Model file for the job. Use its own axes, mm. Face numbers are marked on the shaded views. Coordinates: 2 decimals unless noted, no trailing zeros. Order: outer loops, then holes, each group sorted by start corner. A loop starts at its lowest first (then second) coordinate and runs counter-clockwise, first axis right, second up.
from build123d import *

# Parameters (mm, degrees)
F0_R     = 27
F0_R_2   = 24.925
F1_DEPTH = 13
F0_R_3   = 22.25
F2_DEPTH = 3.5
F3_START = 2.3
F0_R_4   = 27.825
F3_DEPTH = 8.7
F4_SIZE  = 0.3
F5_SIZE  = 0.75


with BuildPart() as f1:
    # F0 (on Top) → F1 (new body)
    with BuildSketch(Plane.XY):
        Circle(F0_R)
        Circle(F0_R_2, mode=Mode.SUBTRACT)
    extrude(amount=F1_DEPTH)

    # F0 (on Top) → F2 (join)
    with BuildSketch(Plane.XY):
        Circle(F0_R_2)
        Circle(F0_R_3, mode=Mode.SUBTRACT)
    extrude(amount=F2_DEPTH)

    # F0 (on Top) → F3 (join)
    with BuildSketch(Plane.XY.offset(F3_START)):
        Circle(F0_R_4)
        Circle(F0_R, mode=Mode.SUBTRACT)
    extrude(amount=F3_DEPTH)

    # F4
    f4_edges = [f1.edges().sort_by_distance(p)[0] for p in [
        (-27, 0, 13),
        (-27, 0, 0),
    ]]
    chamfer(f4_edges, length=F4_SIZE)

    # F5
    f5_edges = [f1.edges().sort_by_distance(p)[0] for p in [
        (27.825, 0, 6.65),
        (-27.825, 0, 2.3),
        (-27.825, 0, 11),
    ]]
    chamfer(f5_edges, length=F5_SIZE)


solid = f1.part
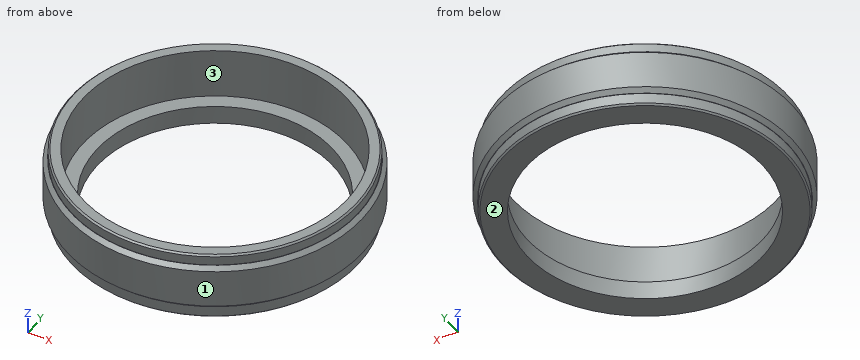
Q1. Mould opens along Y. For the marked faces 1, 2 and 3 say: pulls with the +Y half, pulls with the -Y half, needs draft (parallel to the pull), parting line crosses it, or undercut.
Established:
face 1: parting line crosses it
face 2: needs draft
face 3: undercut
Q2. Probe line 1 (Y direction, x = 0, z = 1.35); line 2 (Y direction, x = 0, z = 8.75) (3 decimals); line 3 (X direction, y = 0.5, z = 9). List the from-to ranges inside material, lowest first.
Established:
line 1: y = -27 to -22.25, 22.25 to 27
line 2: y = -27.825 to -24.925, 24.925 to 27.825
line 3: x = -27.82 to -24.92, 24.92 to 27.82
Q3. Cut at A-A, the plane x = 0. List the corners of the cut face in (y, z) (3 decimals).
Established:
outline: (-27.825, 3.05) - (-27.075, 2.3) - (-27, 2.3) - (-27, 0.3) - (-26.7, 0) - (-22.25, 0) - (-22.25, 3.5) - (-24.925, 3.5) - (-24.925, 13) - (-26.7, 13) - (-27, 12.7) - (-27, 11) - (-27.075, 11) - (-27.825, 10.25) - close; (22.25, 0) - (26.7, 0) - (27, 0.3) - (27, 2.3) - (27.075, 2.3) - (27.825, 3.05) - (27.825, 10.25) - (27.075, 11) - (27, 11) - (27, 12.7) - (26.7, 13) - (24.925, 13) - (24.925, 3.5) - (22.25, 3.5) - close
Q4. Drop flat-ended pins along their axis: P1, Ø5, axis at x = 15, z = 3.5, coming from the -Y side; P2, Ø5, axis at x = 18.5, z = 4.5, coming from the -Y side; P3, Ø5, axis at x = 6, y = -18.5, coming from the +Z side; P4, Ø4, axis at y = -3.5, z = 2.5, coming from the -X side. Give the stop position or say it passes through.
Established:
P1: stops at y = -24.86
P2: stops at y = -22.76
P3: passes through
P4: stops at x = -27.78
Q5. Cut at C-C, the plane z = 5.25. List the corners of the cut face in (x, y) (3 decimals).
Established:
outline: circle Ø55.65 at (0, 0); hole circle Ø49.85 at (0, 0)
